Here's how the part is built. I have some questions about the finished solid (model axes, mm). A direction names the side the tool comes from. Give positions to 0.01 mm unless a question says otherwise; leave off trailing zeros. Write each loop counter-clockwise with the first axis right and the second up, starting at its lowest first coordinate (ties: lowest second). Pieces come first, ordered by that corner, then holes. Notation, with made-up numbers: (-34.75, -36.75) - (4.25, -36.75) arc R19 cw to (4.25, -30.75) - close; hole circle Ø2 at (85.25, 34.5). An arc over 180 degrees is marked (long way). Use a Markdown table: item, result.
```python
from build123d import *

# Parameters (mm, degrees)
F1_DEPTH       = 4.7625
F3_DEPTH       = 127
F5_DEPTH       = 6.35
F7_DEPTH       = 12.7
F9_DEPTH       = 5.08
F11_ANGLE_BACK = 20
F11_ANGLE      = 40
F12_R          = 5.08


# Not quite as in the source:
# - a length typed as a fraction of an inch, garbled in the dataset ("3 / 203.2 mm" for 3/8 in), is restored
# - a pattern or mirror of a feature is missing from the dataset's text; its kind, count and spacing are read off the source's solid


with BuildPart() as f1:
    # F0 (on Top) → F1 (new body)
    with BuildSketch(Plane.XY):
        with BuildLine():
            ThreePointArc((-76.2, 0), (0, -76.2), (76.2, 0))
            Line((76.2, 0), (67.31, 0))
            Line((67.31, 0), (67.31, -12.7))
            Line((67.31, -12.7), (-67.31, -12.7))
            Line((-67.31, -12.7), (-67.31, 0))
            Line((-67.31, 0), (-76.2, 0))
        make_face()
    extrude(amount=F1_DEPTH)

    # F2 (on face) → F3 (join)
    with BuildSketch(Plane.XY.offset(4.7625)):
        with BuildLine():
            Line((-67.31, 0), (-76.2, 0))
            ThreePointArc((-76.2, 0), (0, -76.2), (76.2, 0))
            Line((76.2, 0), (67.31, 0))
            ThreePointArc((67.31, 0), (0, -67.31), (-67.31, 0))
        make_face()
    extrude(amount=F3_DEPTH)

    # F4 (on face) → F5 (join)
    with BuildSketch(Plane.XY.offset(131.7625)):
        with BuildLine():
            Line((76.2, 0), (-76.2, 0))
            ThreePointArc((-76.2, 0), (0, -76.2), (76.2, 0))
        make_face()
    extrude(amount=F5_DEPTH)

    # F6 (on face) → F7 (join)
    with BuildSketch(Plane.XY.offset(138.1125)):
        Polygon((12.7, -14.0898204726), (0, -14.0898204726), (-12.7, -14.0898204726), (-12.7, -19.1698204726), (0, -19.1698204726), (12.7, -19.1698204726), align=None)
    extrude(amount=F7_DEPTH)

    # F8 (on face) → F9 (join)
    with BuildSketch(Plane.YZ.offset(12.7)):
        Polygon((-19.1698204726, 150.8125), (-26.7898204726, 138.1125), (-19.1698204726, 138.1125), align=None)
    f9 = extrude(amount=-F9_DEPTH)

    # F9_copies: F9 across plane
    add(f9.mirror(Plane(origin=(0, 0, 0), x_dir=(0, 0, -1), z_dir=(-1, 0, 0))))


with BuildPart() as f11:
    # F10 (on Right) → F11 (revolve)
    with BuildSketch(Plane.YZ, mode=Mode.PRIVATE) as f11_sk:
        Polygon((-98.6883191255, -24.4902079291), (-69.5020258427, 0), (-76.2, 0), (-76.2, 5.1620067097), (-104.2903103798, -17.814014726), align=None)
    revolve(f11_sk.sketch.rotate(Axis((0, 0, 0), (0, 0, -1)), -F11_ANGLE_BACK), axis=Axis((0, 0, 0), (0, 0, -1)), revolution_arc=F11_ANGLE)

    # F12
    f12_edges = [f11.edges().sort_by_distance(p)[0] for p in [
        (34.71139, -95.36876, -21.152111),
        (-34.71139, -95.36876, -21.152111),
    ]]
    fillet(f12_edges, radius=F12_R)


solid = f1.part
```
Item 1: I need wall thicknesses on line 1 along Z through (x, y) = (39, -34); line 2 along X through (y, z) = (-51, 116.5); line 3 along X through (y, z) = (-40, 77.5). Which ranges of each line are inside material? Lowest first, please. Write a range as [from, to].
Values:
| item | result |
|---|---|
| line 1 | z = [0, 4.76], [131.76, 138.11] |
| line 2 | x = [-56.62, -43.93], [43.93, 56.62] |
| line 3 | x = [-64.86, -54.14], [54.14, 64.86] |
Item 2: For faces 4 (the flat face through (7.62, -21, 142)), 5 (the flat face through (1, -12.7, 2)), 6 (the flat face through (0, -14.09, 144)), 7 (the flat face through (12.7, -19, 143)), 8 (the cylindrical face through (1.48, -67.294, 67.374)), which set-ups out of +Z, -Z, +X, -X, +Y, -Y let a thin tool reach every point of the face, with its end or its side?
Values:
| item | result |
|---|---|
| face 4 | +Z, -Y |
| face 5 | -Z, +Y |
| face 6 | +Z, +X, -X, +Y |
| face 7 | +Z, +X, +Y, -Y |
| face 8 | +Y |
Item 3: Will these pins go through, and if not, where does the flat tip stop? pin 1 Ø4 at (y, z) = (-22.5, 146) entering from -X; pin 2 Ø2 at (y, z) = (-30, 134.5) entering from +X; pin 3 Ø4 at (y, z) = (-21.5, 141.5) entering from +X.
Values:
| item | result |
|---|---|
| pin 1 | stops at x = -12.7 |
| pin 2 | stops at x = 70.47 |
| pin 3 | stops at x = 12.7 |
Item 4: If we section it at C-C, the plane z = 95: Write out the boundary of the cut face in (x, y).
Values:
| item | result |
|---|---|
| outline | (-76.2, 0) arc R76.2 ccw to (76.2, 0) - (67.31, 0) arc R67.31 cw to (-67.31, 0) - close |
Item 5: If we section it at B-B, the plane x = 0: Write out the boundary of the cut face in (y, z).
Values:
| item | result |
|---|---|
| outline | (-76.2, 0) - (-12.7, 0) - (-12.7, 4.76) - (-67.31, 4.76) - (-67.31, 131.76) - (0, 131.76) - (0, 138.11) - (-14.09, 138.11) - (-14.09, 150.81) - (-19.17, 150.81) - (-19.17, 138.11) - (-76.2, 138.11) - close |
Item 6: Thinking about a two-plate mould opening in X: for faces 1 (the flat face through (0, -19.17, 144)), 2 (the flat face through (-1, -38, 0)), 3 (the flat face through (-12.7, -19, 143)), which applies, +X half, -X half, draft (parallel to the pull), parting line (faces both ways), or undercut?
Values:
| item | result |
|---|---|
| face 1 | undercut |
| face 2 | draft |
| face 3 | -X half |
Item 7: If we section it at D-D, the plane y = -5: Write out the boundary of the cut face in (x, z), plus the area to 3 significant figures.
Values:
| item | result |
|---|---|
| outline | (-76.04, 0) - (-67.31, 0) - (-67.31, 4.76) - (-67.12, 4.76) - (-67.12, 131.76) - (67.12, 131.76) - (67.12, 4.76) - (67.31, 4.76) - (67.31, 0) - (76.04, 0) - (76.04, 138.11) - (-76.04, 138.11) - close |
| area | 3,310 mm2 |
Item 8: If we section it at A-A, the plane y = -64: Write out the boundary of the cut face in (x, z), plus the area to 3 significant figures.
Values:
| item | result |
|---|---|
| outline | (-41.36, 0) - (41.36, 0) - (41.36, 138.11) - (-41.36, 138.11) - close; hole (-20.85, 4.76) - (20.85, 4.76) - (20.85, 131.76) - (-20.85, 131.76) - close |
| area | 6,130 mm2 |
